Autodesk Inventor part; units mm, degrees
ref_plane "YZ Plane" through (0, 0, 0) normal (1, 0, 0) x (0, 1, 0)
ref_plane "XZ Plane" through (0, 0, 0) normal (0, 1, 0) x (-1, 0, 0)
ref_plane "XY Plane" through (0, 0, 0) normal (0, 0, 1) x (1, 0, 0)
sketch "Skizze3" plane through (0, 0, 0) normal (0, 0, 1) x (1, 0, 0)
  line L0 (-170, 0) -> (170, 0)
  line L1 (170, 0) -> (170, 104)
  line L2 (170, 104) -> (-170, 104)
  line L3 (-170, 104) -> (-170, 0)
  point P0 (0, 0)
  dimension "d3" = 340
  dimension "d4" = 104
extrude "Extrusion1" add sketch "Skizze3" along normal mid plane 202
sketch "Skizze4" plane through (-170, 104, 101) normal (0, 1, 0) x (1, 0, 0)
  line L0 (15, 15) -> (325, 15)
  line L1 (325, 15) -> (325, 187)
  line L2 (325, 187) -> (15, 187)
  line L3 (15, 187) -> (15, 15)
  point P0 (170, 101)
  dimension "d7" = 310
  dimension "d8" = 172
extrude "Extrusion2" cut sketch "Skizze4" against normal blind 91
properties part number "wassertank"
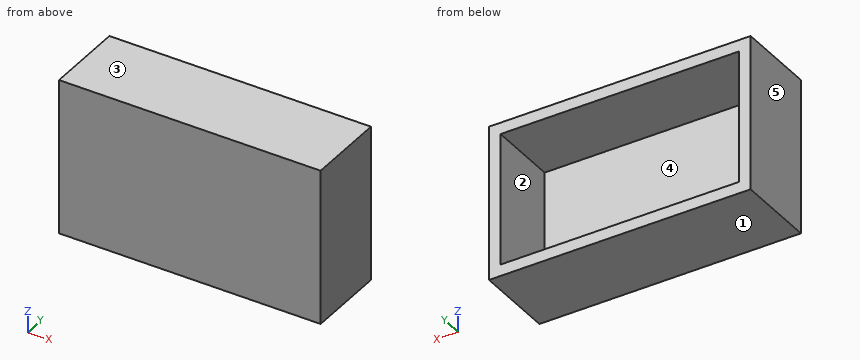
Model file for the job. Use its own axes, mm. Face numbers are marked on the shaded views. A direction names the side the tool comes from. Round coordinates to 2 decimals unless told otherwise and drop trailing zeros. Loops run counter-clockwise (first coordinate to the right, second up) from the corner with the lowest first, then second, coordinate; pieces in that order, holes last. Notation, with made-up numbers: M 8,58.25 L 15,58.25 A13 cw 15,83.25 Z; hole C 57,-9.75 d10. An arc over 180 degrees is marked long. One line per question, with ' | ' between items.
1) Band-saw the part on C-C (x = 72.5). Give the cut face in (y, z), then the cut area to 3 significant figures.
Solved:
outline: M 0,-101 L 104,-101 L 104,-86 L 13,-86 L 13,86 L 104,86 L 104,101 L 0,101 Z | area: 5,360 mm²
2) Mould opens along X. For the marked faces 3, 4 and 5 say: +X half, -X half, draft (parallel to the pull), parting line (faces both ways), or undercut.
Solved:
face 3: draft | face 4: undercut | face 5: -X half
3) Band-saw the part on B-B (z = -39). Give the cut face in (x, y).
Solved:
outline: M -170,0 L 170,0 L 170,104 L 155,104 L 155,13 L -155,13 L -155,104 L -170,104 Z
4) Drill centre lines: line 1 along Z through (x, y) = (-153, 18); line 2 along X through (y, z) = (95, 10); line 3 along Y through (x, z) = (135.5, -40.5). Where is each one in solid material? Low to high.
Solved:
line 1: z = -101 to -86, 86 to 101 | line 2: x = -170 to -155, 155 to 170 | line 3: y = 0 to 13
5) Band-saw the part on A-A (y = 75). Give the cut face in (x, z), then the cut area to 3 significant figures.
Solved:
outline: M -170,-101 L 170,-101 L 170,101 L -170,101 Z; hole M -155,-86 L 155,-86 L 155,86 L -155,86 Z | area: 15,400 mm²
6) Flat gauge pin, fed straight in: pin 1 (3 mm diameter, centred on x = 68, z = 76.5, fed in from +Y). Where does the tip first touch, or does it go through?
Solved:
pin 1: stops at y = 13
7) 3-axis set-ups, long thin cutter, end or side, ignore diameter. For the marked faces 1 and 2: which of +Z, -Z, +X, -X, +Y, -Y reach the whole face in a straight line?
Solved:
face 1: -Z, +X, -X, +Y, -Y | face 2: +Y
